Design review of the part shown in the three views and the two pictorial views. Dimensions are in mm from the part's minimum x, y and z. Coordinates: 2 decimals unless noted, no trailing zeros. Loops run counter-clockwise (first coordinate to the right, second up) from the corner with the lowest first, then second, coordinate; pieces in that order, holes last. Notation, with made-up numbers: (62, 38) - (73, 38) arc R10 cw to (73, 47) - close; hole circle Ø5 at (66.25, -15). An arc over 180 degrees is marked (long way). One line per item, written item: value. Start each with the question number.
1. Take a section at C-C, the plane x = 45. State the section outline as (y, z) points (1 decimal).
2. Take a section at A-A, the plane y = 20. State the section outline as (x, z) points, and give its area (3 significant figures).
3. To check wall thickness, follow line 1 (X direction, y = 79, z = 1.25); line 2 (Y direction, x = 32, z = 1.2) (1 decimal); line 3 (Y direction, x = 45, z = 1.5) (1 decimal). State the ranges of each line that lie inside material, in increasing order. Write a range as from..to.
4. Take a section at B-B, the plane z = 0.75. State the section outline as (x, y) points (1 decimal).
5. Take a section at D-D, the plane y = 97. State the section outline as (x, z) points.
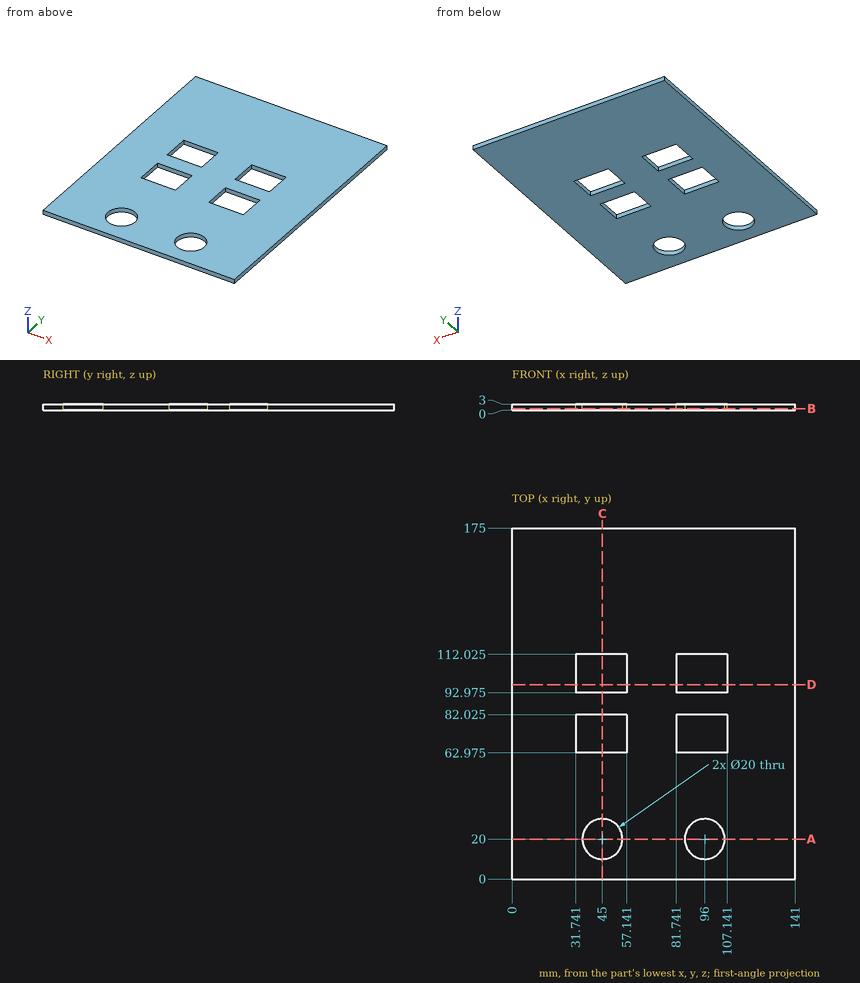
Solutions:
1. outline: (0, 0) - (10, 0) - (10, 3) - (0, 3) - close; (30, 0) - (63, 0) - (63, 3) - (30, 3) - close; (82, 0) - (93, 0) - (93, 3) - (82, 3) - close; (112, 0) - (175, 0) - (175, 3) - (112, 3) - close
2. outline: (0, 0) - (35, 0) - (35, 3) - (0, 3) - close; (55, 0) - (86, 0) - (86, 3) - (55, 3) - close; (106, 0) - (141, 0) - (141, 3) - (106, 3) - close
2. area: 303 mm2
3. line 1: 0..31.74, 57.14..81.74, 107.14..141
3. line 2: 0..63, 82..93, 112..175
3. line 3: 0..10, 30..63, 82..93, 112..175
4. outline: (0, 0) - (141, 0) - (141, 175) - (0, 175) - close; hole (31.7, 63) - (57.1, 63) - (57.1, 82) - (31.7, 82) - close; hole (31.7, 93) - (57.1, 93) - (57.1, 112) - (31.7, 112) - close; hole circle Ø20 at (45, 20); hole (81.7, 63) - (107.1, 63) - (107.1, 82) - (81.7, 82) - close; hole (81.7, 93) - (107.1, 93) - (107.1, 112) - (81.7, 112) - close; hole circle Ø20 at (96, 20)
5. outline: (0, 0) - (31.74, 0) - (31.74, 3) - (0, 3) - close; (57.14, 0) - (81.74, 0) - (81.74, 3) - (57.14, 3) - close; (107.14, 0) - (141, 0) - (141, 3) - (107.14, 3) - close
